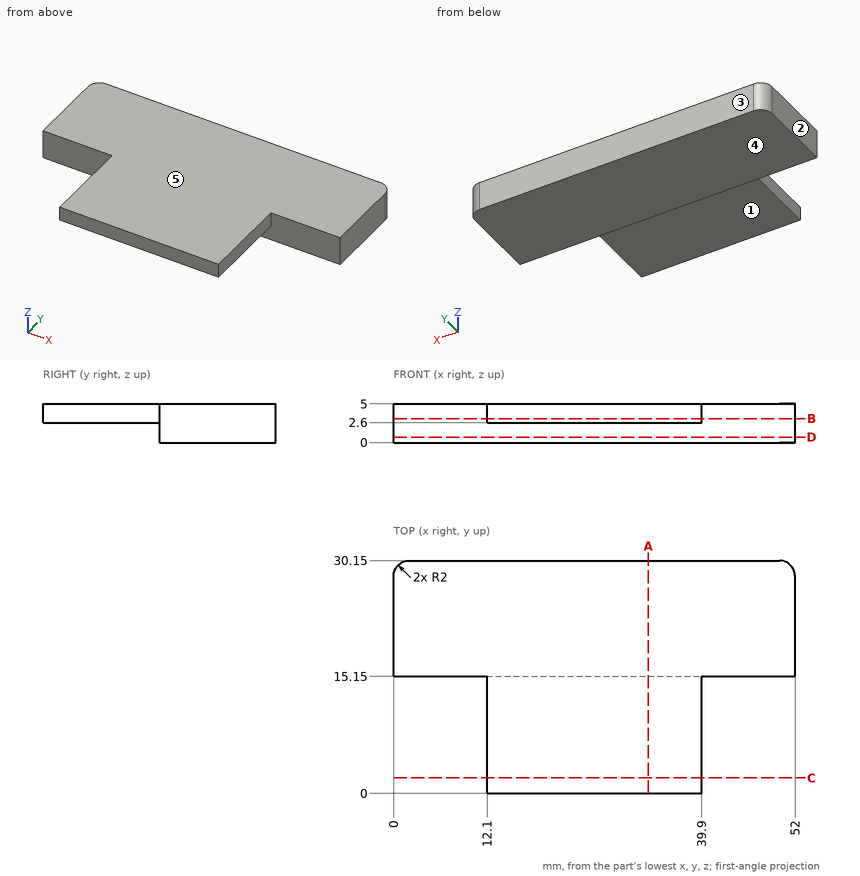
Could you check a few things on this drawing? It's one solid part, dimensions in mm from its lowest x, y, z. A direction names the side the tool comes from. Coordinates: 2 decimals unless noted, no trailing zeros. Write each loop counter-clockwise with the first axis right and the second up, starting at its lowest first coordinate (ties: lowest second). Pieces come first, ordered by that corner, then holes. Notation, with made-up numbers: M -29,11 L 2,11 A17 cw 2,24 Z; hole C -33,-32 d5. An arc over 180 degrees is marked long. Answer as CSV lines item,"result". Start each with the question number.
Q1. Suppose I cut it at C-C, the plane y = 2. List the corners of the cut face in (x, z) for me, then the cut area to 3 significant figures.
Q2. If we mould it in two halves opening along Z, with no side actions, what happens to the marked faces 3, 4 and 5? For each: pulls with the +Z half, pulls with the -Z half, needs draft (parallel to the pull), parting line crosses it, or undercut.
Q3. Will these pins go through, and if not, where does the flat tip stop? pin 1 Ø4.5 at (x, y) = (20, 10.5) entering from -Z; pin 2 Ø2.5 at (y, z) = (11, 4) entering from +X; pin 3 Ø1.5 at (x, z) = (12, 0.5) entering from -Y.
Q4. Suppose I cut it at D-D, the plane z = 0.7. List the corners of the cut face in (x, y) for me, then the cut area to 3 significant figures.
Q5. Suppose I cut it at A-A, the plane x = 33. List the corners of the cut face in (y, z) for me.
Q6. I need wall thicknesses on probe 1 along Y at (x, z) = (8, 2.95); probe 2 along X at (y, z) = (8.5, 4.05); probe 3 along Z at (x, y) = (16.5, 12). Which ranges of each line are inside material? Lowest first, please. Write a range as [from, to].
Q7. Suppose I cut it at B-B, the plane z = 3.1. List the corners of the cut face in (x, y) for me, then the cut area to 3 significant figures.
Q8. For the marked faces 1 and 2, which set-ups out of +Z, -Z, +X, -X, +Y, -Y let a thin tool reach every point of the face, with its end or its side?
Entries:
1,outline,"M 12.1,2.6 L 39.9,2.6 L 39.9,5 L 12.1,5 Z"
1,area,"66.7 mm²"
2,face 3,"needs draft"
2,face 4,"pulls with the -Z half"
2,face 5,"pulls with the +Z half"
3,pin 1,"stops at z = 2.6"
3,pin 2,"stops at x = 39.9"
3,pin 3,"stops at y = 15.15"
4,outline,"M 0,15.15 L 52,15.15 L 52,28.15 A2 ccw 50,30.15 L 2,30.15 A2 ccw 0,28.15 Z"
4,area,"778 mm²"
5,outline,"M 0,2.6 L 15.15,2.6 L 15.15,0 L 30.15,0 L 30.15,5 L 0,5 Z"
6,probe 1,"y = [15.15, 30.15]"
6,probe 2,"x = [12.1, 39.9]"
6,probe 3,"z = [2.6, 5]"
7,outline,"M 0,15.15 L 12.1,15.15 L 12.1,0 L 39.9,0 L 39.9,15.15 L 52,15.15 L 52,28.15 A2 ccw 50,30.15 L 2,30.15 A2 ccw 0,28.15 Z"
7,area,"1,200 mm²"
8,face 1,"-Z, +X, -X, -Y"
8,face 2,"+Z, -Z, -X, +Y, -Y"
